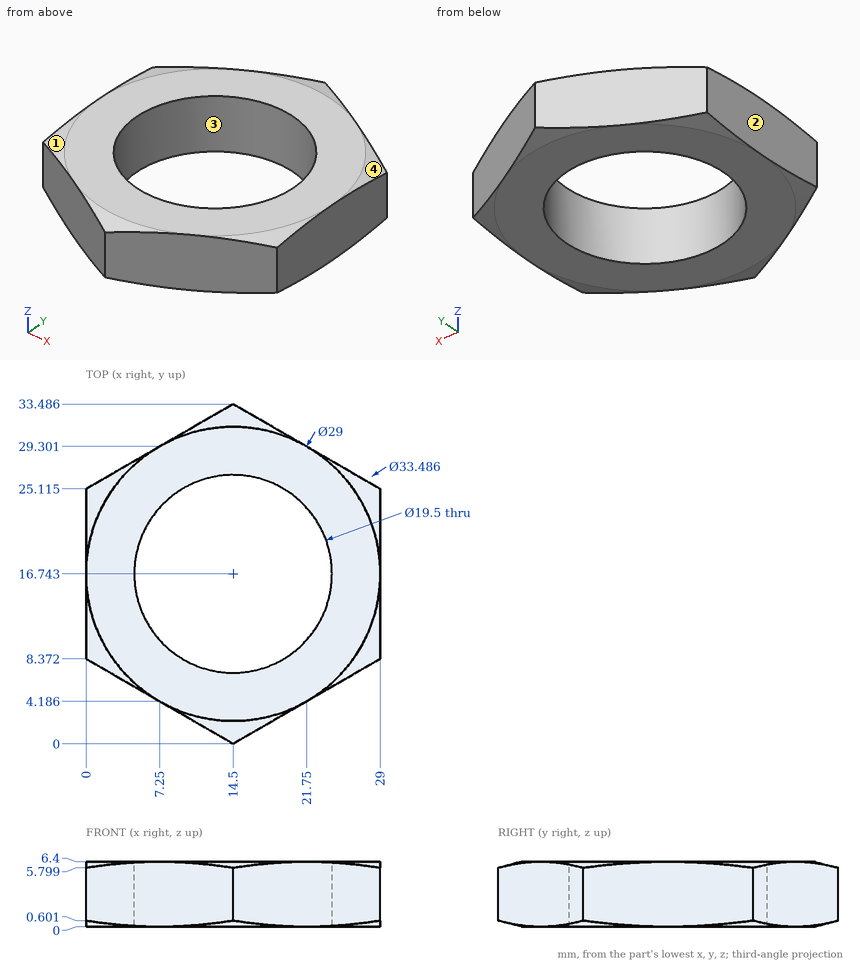
The figure shows three views and two pictorial views of one solid part (mm, origin at its lowest corner). Answer the questions. Coordinates: 2 decimals unless noted, no trailing zeros.
1. For a pull along Y with two mould halves and no side action, classify the marked faces 1, 2, 3 and 4 as +Y half, -Y half, draft (parallel to the pull), parting line (faces both ways), or undercut.
Results list:
face 1: -Y half
face 2: draft
face 3: undercut
face 4: +Y half
2. Consider line 1 along X through (y, z) = (22, 5.5); line 2 along Y through (x, z) = (16.5, 4.5) (1 decimal); line 3 along X through (y, z) = (11, 2). Determine where each line is inside the solid, lowest interval first.
Results list:
line 1: x = 0 to 6.29, 22.71 to 29
line 2: y = 1.2 to 7.2, 26.3 to 32.3
line 3: x = 0 to 6.62, 22.38 to 29
3. Flat-ended cylindrical pins translate along their axes: pin 1 (1 mm diameter, centred on x = 21, z = 1, fed in from +Y); pin 2 (3 mm diameter, centred on x = 8.5, y = 3.5, fed in from +Z); pin 3 (1.5 mm diameter, centred on x = 24.5, z = 5, fed in from -Y); pin 4 (1.5 mm diameter, centred on x = 20, z = 1, fed in from -Y). Find the tip coordinate at first contact, or state that the pin passes through.
Results list:
pin 1: stops at y = 30.02
pin 2: stops at z = 6.4
pin 3: stops at y = 5.34
pin 4: stops at y = 2.74
